Geometry check sheet. Reference: the model listing, model coordinates, mm. Give positions to 0.01 mm unless a question says otherwise; leave off trailing zeros. Write each loop counter-clockwise with the first axis right and the second up, starting at its lowest first coordinate (ties: lowest second). Pieces come first, ordered by that corner, then holes. Notation, with made-up numbers: M -23.5,-24 L 9.5,-24 A6 ccw 9.5,-18 Z; hole C 59,33 d5. An arc over 180 degrees is marked long. Write each question's results on one line, items separated by ' | '.
Solid Edge part; units mm, degrees
sketch "Sketch1" plane through (0, 0, 0) normal (0, 0, 1) x (1, 0, 0)
  line L0 (-53.9742, 23.7118) -> (53.9742, 23.7118)
  line L1 (-31.7069, -8.1496) -> (31.7069, -8.1496)
  arc A0 (-31.7069, -8.1496) -> (-53.9742, 23.7118) centre (-53.9742, 0) cw
  arc A1 (53.9742, 23.7118) -> (31.7069, -8.1496) centre (53.9742, 0) cw
extrude "Protrusion1" add sketch "Sketch1" along normal mid plane 55
fillet "Round_1" radius 12 2 edges at (-31.7069, -8.1496, 0) (31.7069, -8.1496, 0)
draft "Draft1" angle 10 neutral plane through (0, 0, 27.5) normal (0, 0, 1) pull direction (0, 0, -1) face at (-37.0623, 23.7118, 17.7833) face at (-16.8164, -8.1496, 17.7833) face at (-46.3591, -22.4557, 17.7833) face at (-33.2565, -11.9553, -17.7833) face at (68.2174, 18.9573, 17.7833) face at (33.2565, -11.9553, 17.7833)
Q1. Release check for a two-part mould opening along X. For faces 1 (the face through (-0.756, 18.795, -0.385)), 2 (the face through (-0.343, -3.233, -0.385)) record: released by +X, released by -X, zero draft, split by the parting line, or undercut.
Answer key:
face 1: zero draft | face 2: undercut
Q2. Section check A-A (z = 21.5). Enter the section's corners in (x, y).
Answer key:
outline: M -53.97,22.65 A22.65 ccw long -35.27,-12.78 A13.06 cw -24.49,-7.09 L 24.49,-7.09 A13.06 cw 35.27,-12.78 A22.65 ccw long 53.97,22.65 Z
Q3. Section check C-C (z = -4.5). Enter the section's corners in (x, y), then the cut area to 3 significant figures.
Answer key:
outline: M -53.97,18.07 A18.07 ccw long -39.06,-10.2 A17.64 cw -24.49,-2.51 L 24.49,-2.51 A17.64 cw 39.06,-10.2 A18.07 ccw long 53.97,18.07 Z | area: 3,710 mm2
Q4. Depth check by flat-ended pin: P1, Ø10, axis at y = 2, z = 17, coming from the +X side; P2, Ø4, axis at x = 38.5, z = 14, coming from the -Y side; P3, Ø4, axis at y = 5.5, z = 8.5, coming from the +X side. Enter the tip coordinate at first touch or a pass-through.
Answer key:
P1: stops at x = 76.68 | P2: stops at y = -16.6 | P3: stops at x = 74.18
Q5. Section check B-B (x = -3.5). Enter the section's corners in (y, z).
Answer key:
outline: M -8.15,27.5 L 1.55,-27.5 L 14.01,-27.5 L 23.71,27.5 Z
Q6. Material ranges on probe 1 along X at (y, z) = (-7, -10); probe 2 along X at (y, z) = (-12.5, -16); probe 3 along X at (y, z) = (-2, -4), recorded low to high. Write a range as [from, to].
Answer key:
probe 1: x = [-69.58, -37.66], [37.66, 69.58] | probe 2: x = [-64.03, -43.92], [43.92, 64.03] | probe 3: x = [-72.02, 72.02]
